Verification items for this drawing (mm, ordinates from the low corner). A direction names the side the tool comes from. Give positions to 0.01 mm unless a question says otherwise; leave off trailing zeros. Loops run counter-clockwise (first coordinate to the right, second up) from the corner with the lowest first, then second, coordinate; pieces in that order, holes last. Notation, with made-up numbers: M 2,-36.75 L 50,-36.75 A14 ccw 50,-23.75 Z; hole C -26.75,47 d6. An arc over 180 degrees is marked long. Use a Markdown table: item, result.
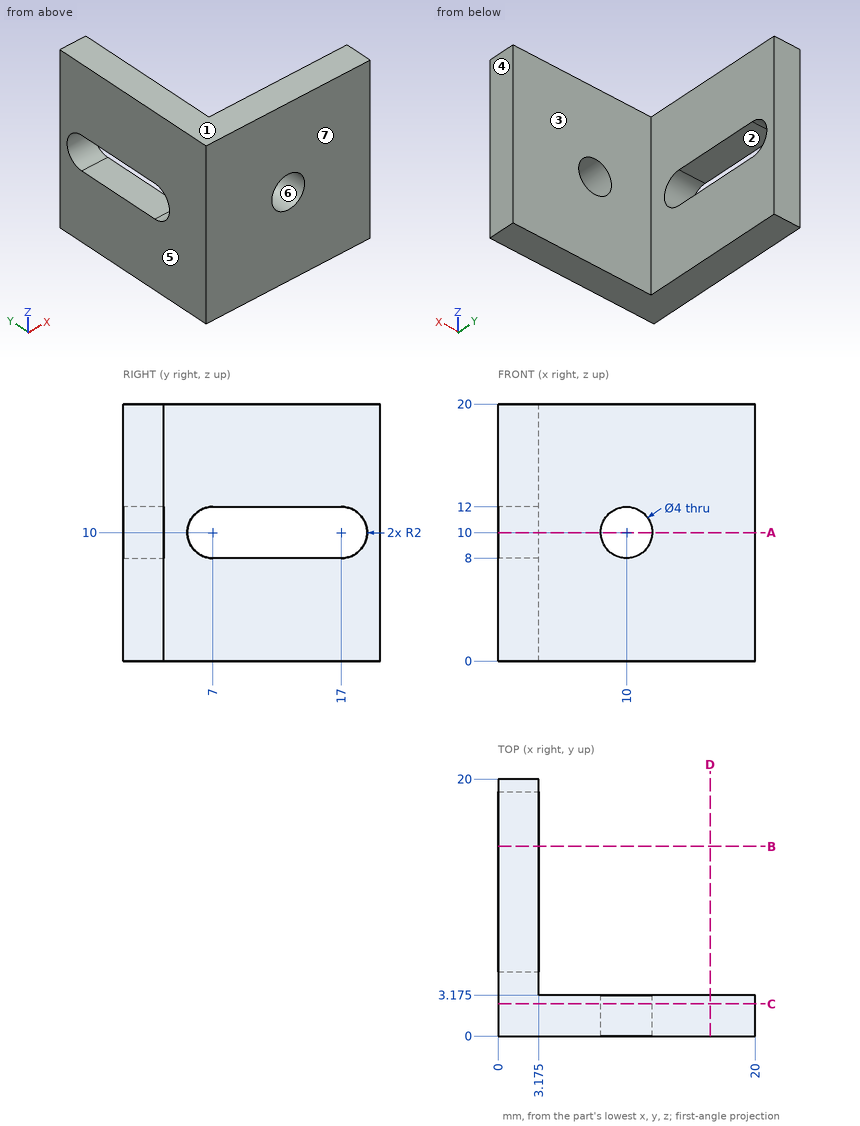
(1) Draft check along X on the marked faces 4, 5, 6 and 7. Enter one of: +X half, -X half, draft (parallel to the pull), parting line (faces both ways), or undercut.
Results below:
| item | result |
|---|---|
| face 4 | +X half |
| face 5 | -X half |
| face 6 | undercut |
| face 7 | draft |
(2) Cross-section at C-C on y = 2.5. Record the cut outline in (x, z).
Results below:
| item | result |
|---|---|
| outline | M 0,0 L 20,0 L 20,20 L 0,20 Z; hole C 10,10 d4 |
(3) Set-up check for the marked faces 1, 2 and 3: record each of +Z, -Z, +X, -X, +Y, -Y from which the full face is reachable in a straight line by a thin tool's end or side.
Results below:
| item | result |
|---|---|
| face 1 | +Z, +X, -X, +Y, -Y |
| face 2 | +X, -X |
| face 3 | +Z, -Z, +X, +Y |
(4) Cross-section at A-A on z = 10. Record the cut outline in (x, y) (3 decimals).
Results below:
| item | result |
|---|---|
| outline | M 0,0 L 8,0 L 8,3.175 L 3.175,3.175 L 3.175,5 L 0,5 Z; M 0,19 L 3.175,19 L 3.175,20 L 0,20 Z; M 12,0 L 20,0 L 20,3.175 L 12,3.175 Z |
(5) Cross-section at D-D on x = 16.5. Record the cut outline in (y, z) (3 decimals).
Results below:
| item | result |
|---|---|
| outline | M 0,0 L 3.175,0 L 3.175,20 L 0,20 Z |
(6) Cross-section at B-B on y = 14.75. Record the cut outline in (x, z) (3 decimals).
Results below:
| item | result |
|---|---|
| outline | M 0,0 L 3.175,0 L 3.175,8 L 0,8 Z; M 0,12 L 3.175,12 L 3.175,20 L 0,20 Z |
(7) Gauge pin test, flat ends, axial feed: P1, Ø8.5, axis at y = 11.5, z = 5.5, coming from the +X side (3 decimals); P2, Ø4.5, axis at x = 10, z = 10, coming from the +Y side (3 decimals). Record the tip position at first contact, or that the pin passes through.
Results below:
| item | result |
|---|---|
| P1 | x = 3.175 |
| P2 | y = 3.175 |
(8) Material ranges on line 1 (X direction, y = 1.8, z = 10); line 2 (Y direction, x = 18.5, z = 6.5) (3 decimals), recorded low to high.
Results below:
| item | result |
|---|---|
| line 1 | 0 to 8, 12 to 20 |
| line 2 | 0 to 3.175 |
